from build123d import *

# Parameters (mm, degrees)
SKETCH1_W           = 100
SKETCH1_H           = 254
BOSS_EXTRUDE1_DEPTH = 3
SKETCH2_W           = 50
SKETCH2_H           = 3
BOSS_EXTRUDE2_DEPTH = 3
SKETCH3_W           = 20
SKETCH3_H           = 3
CUT_EXTRUDE1_DEPTH  = 3
SKETCH4_W           = 3
SKETCH4_H           = 40
SKETCH4_H_2         = 50
BOSS_EXTRUDE3_DEPTH = 3
SKETCH5_W           = 20
SKETCH5_H           = 3
CUT_EXTRUDE2_DEPTH  = 3


with BuildPart() as part:
    # Sketch1 → Boss-Extrude1 (new body)
    with BuildSketch(Plane.XY):
        with Locations((-9.252144082, -28.319039451)):
            Rectangle(SKETCH1_W, SKETCH1_H)
    extrude(amount=BOSS_EXTRUDE1_DEPTH)

    # Sketch2 → Boss-Extrude2 (add)
    with BuildSketch(Plane.XZ.offset(155.319039451)):
        with Locations((-9.252144082, 1.5)):
            Rectangle(SKETCH2_W, SKETCH2_H)
    extrude(amount=BOSS_EXTRUDE2_DEPTH)

    # Sketch3 → Cut-Extrude1 (cut)
    with BuildSketch(Plane(origin=(0, 98.680960549, 0), x_dir=(1, 0, 0), z_dir=(0, 1, 0))):
        with Locations((-29.252144082, -1.5)):
            Rectangle(SKETCH3_W, SKETCH3_H)
        with Locations((10.747855918, -1.5)):
            Rectangle(SKETCH3_W, SKETCH3_H)
    extrude(amount=-CUT_EXTRUDE1_DEPTH, mode=Mode.SUBTRACT)

    # Sketch4 → Boss-Extrude3 (add)
    with BuildSketch(Plane(origin=(40.747855918, 0, 0), x_dir=(0, 0, -1), z_dir=(1, 0, 0))):
        with Locations((-1.5, -115.319039451)):
            Rectangle(SKETCH4_W, SKETCH4_H)
        with Locations((-1.5, -23.319039451)):
            Rectangle(SKETCH4_W, SKETCH4_H)
        with Locations((-1.5, 73.680960549)):
            Rectangle(SKETCH4_W, SKETCH4_H_2)
    extrude(amount=BOSS_EXTRUDE3_DEPTH)

    # Sketch5 → Cut-Extrude2 (cut)
    with BuildSketch(Plane(origin=(0, 0, 0), x_dir=(-1, 0, 0), z_dir=(0, 0, -1))):
        with Locations((-10.747855918, -68.819039451)):
            Rectangle(SKETCH5_W, SKETCH5_H)
        with Locations((34.252144082, -68.819039451)):
            Rectangle(SKETCH5_W, SKETCH5_H)
    extrude(amount=-CUT_EXTRUDE2_DEPTH, mode=Mode.SUBTRACT)


solid = part.part
Part model, mm, in its own coordinate system. Coordinates: 2 decimals unless noted, no trailing zeros. Write each loop counter-clockwise with the first axis right and the second up, starting at its lowest first coordinate (ties: lowest second). Pieces come first, ordered by that corner, then holes. Notation, with made-up numbers: M 46,-3 L 51,-3 A23 cw 51,6 Z; hole C -33.75,45 d2. An arc over 180 degrees is marked long. Return JSON: item names as keys, results as strings.
1. Saw through at C-C, the plane y = 34.5. Write the cut outline in (x, z).
Determined:
{"outline": "M -59.25,0 L 40.75,0 L 40.75,3 L -59.25,3 Z"}
2. Saw through at B-B, the plane z = 1.3. Count the separate pieces of the cut face and the enclosed holes in it, then the cut area to 3 significant figures.
Determined:
{"separate pieces": "1", "enclosed holes": "2", "area": "25,700 mm²"}
3. Probe L1, parallel to Y at x = -30, z = 0.2; L2, parallel to Y at x = -41, z = 1.5; L3, parallel to X at y = -71.5, z = 0.7. List the from-to ranges inside material, lowest first.
Determined:
{"L1": "-158.32 to -70.32, -67.32 to 95.68", "L2": "-155.32 to -70.32, -67.32 to 98.68", "L3": "-59.25 to 40.75"}
4. Saw through at A-A, the plane x = 6. Write the cut outline in (y, z), then the cut area to 3 significant figures.
Determined:
{"outline": "M -158.32,0 L -70.32,0 L -70.32,3 L -158.32,3 Z; M -67.32,0 L 95.68,0 L 95.68,3 L -67.32,3 Z", "area": "753 mm²"}
5. Flat gauge pins, fed straight in: pin 1 Ø5 at (x, y) = (4, -107.5) entering from -Z; pin 2 Ø0.9 at (x, z) = (28.5, 1.5) entering from -Y; pin 3 Ø0.9 at (y, z) = (28.5, 2) entering from +X; pin 4 Ø0.9 at (x, z) = (41.5, 2) entering from -Y. Where does each tip first touch, or does it go through?
Determined:
{"pin 1": "z = 0", "pin 2": "y = -155.32", "pin 3": "x = 40.75", "pin 4": "y = -135.32"}
